```python
from build123d import *

# Parameters (mm, degrees)
BOSS_EXTRUDE1_DEPTH = 1.5
SKETCH2_W           = 28
SKETCH2_H           = 12.5
BOSS_EXTRUDE2_DEPTH = 8.5
SKETCH3_R           = 3
BOSS_EXTRUDE3_DEPTH = 4.5
SKETCH4_W           = 28
SKETCH4_H           = 12.5
BOSS_EXTRUDE4_DEPTH = 19.2
SKETCH5_W           = 3.625016777
SKETCH5_H           = 3.044537311
BOSS_EXTRUDE5_DEPTH = 12.5
BOSS_EXTRUDE7_DEPTH = 4


with BuildPart() as part:
    # Sketch1 → Boss-Extrude1 (new body)
    with BuildSketch(Plane(origin=(0, 0, 0), x_dir=(1, 0, 0), z_dir=(0, 1, 0))):
        with BuildLine():
            Line((20.25, -6.25), (-20.25, -6.25))
            Line((-20.25, -6.25), (-20.25, -1))
            Line((-20.25, -1), (-19.5, -1))
            ThreePointArc((-19.5, -1), (-15.234435563, 0), (-19.5, 1))
            Line((-19.5, 1), (-20.25, 1))
            Line((-20.25, 1), (-20.25, 6.25))
            Line((-20.25, 6.25), (20.25, 6.25))
            Line((20.25, 6.25), (20.25, 1))
            Line((20.25, 1), (19.5, 1))
            ThreePointArc((19.5, 1), (15.234435563, 0), (19.5, -1))
            Line((19.5, -1), (20.25, -1))
            Line((20.25, -1), (20.25, -6.25))
        make_face()
    extrude(amount=BOSS_EXTRUDE1_DEPTH)

    # Sketch2 → Boss-Extrude2 (add)
    with BuildSketch(Plane(origin=(0, 1.5, 0), x_dir=(1, 0, 0), z_dir=(0, 1, 0))):
        Rectangle(SKETCH2_W, SKETCH2_H)
    extrude(amount=BOSS_EXTRUDE2_DEPTH)

    # Sketch3 → Boss-Extrude3 (add)
    with BuildSketch(Plane(origin=(0, 10, 0), x_dir=(1, 0, 0), z_dir=(0, 1, 0))):
        with Locations((7, 0)):
            Circle(SKETCH3_R)
    extrude(amount=BOSS_EXTRUDE3_DEPTH)

    # Sketch4 → Boss-Extrude4 (add)
    with BuildSketch(Plane.XZ):
        Rectangle(SKETCH4_W, SKETCH4_H)
    extrude(amount=BOSS_EXTRUDE4_DEPTH)

    # Sketch5 → Boss-Extrude5 (add)
    with BuildSketch(Plane.XY.offset(6.25)):
        with Locations((15.812508389, -12.601527977)):
            Rectangle(SKETCH5_W, SKETCH5_H)
    extrude(amount=-BOSS_EXTRUDE5_DEPTH)

    # Sketch6 → Boss-Extrude7 (add)
    with BuildSketch(Plane(origin=(17.625016777, 0, 0), x_dir=(0, 0, -1), z_dir=(1, 0, 0))):
        with BuildLine():
            Line((-1.532511857, -12.7778257), (-1.512025454, -12.7778257))
            ThreePointArc((-1.512025454, -12.7778257), (0, -14.123796632), (1.512025454, -12.7778257))
            Line((1.512025454, -12.7778257), (1.532511857, -12.7778257))
            ThreePointArc((1.532511857, -12.7778257), (4.566805966, -12.601527977), (1.532511857, -12.425230254))
            Line((1.532511857, -12.425230254), (1.512025454, -12.425230254))
            ThreePointArc((1.512025454, -12.425230254), (0, -11.079259321), (-1.512025454, -12.425230254))
            Line((-1.512025454, -12.425230254), (-1.532511857, -12.425230254))
            ThreePointArc((-1.532511857, -12.425230254), (-4.566805966, -12.601527977), (-1.532511857, -12.7778257))
        make_face()
    extrude(amount=BOSS_EXTRUDE7_DEPTH)


solid = part.part
```
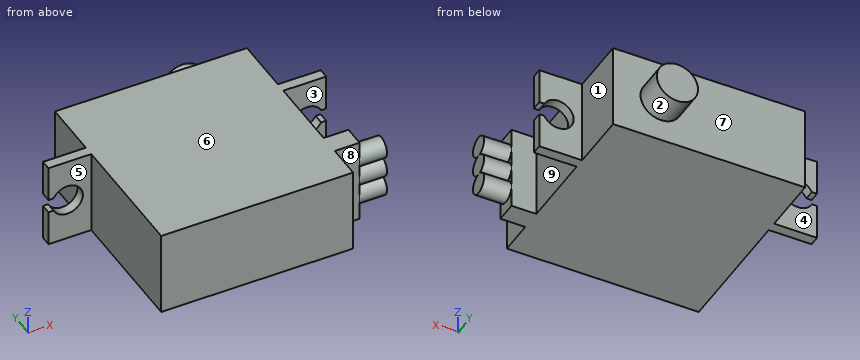
Part model, mm, in its own coordinate system. Face numbers are marked on the shaded views. A direction names the side the tool comes from. Coordinates: 2 decimals unless noted, no trailing zeros. Order: outer loops, then holes, each group sorted by start corner. A loop starts at its lowest first (then second) coordinate and runs counter-clockwise, first axis right, second up. Notation, with made-up numbers: (17.25, 23) -> (55.25, 23) arc R15 cw to (55.25, 42) -> close; hole circle Ø7 at (51.5, 89). An arc over 180 degrees is marked (long way). Put each result on its own line as item: value. Start each with the question number.
(1) Mould opens along Y. For the marked faces 6, 7, 8 and 9 say: pulls with the +Y half, pulls with the -Y half, needs draft (parallel to the pull), parting line crosses it, or undercut.
(2) Band-saw the part on A-A (x = -17.5). Give the cut face in (y, z), then the cut area to 3 significant figures.
(3) Band-saw the part on C-C (x = 17). Give the cut face in (y, z).
(4) Pin check, flat tips, straight feed: pin 1 Ø3 at (x, z) = (16, -3) entering from -Y; pin 2 Ø3 at (x, z) = (18.5, 0.5) entering from +Y; pin 3 Ø3 at (y, z) = (-2.5, -2.5) entering from +X. Stop position of each tip, or through.
(5) Probe line 1 along Y through (x, z) = (17, 5); line 2 along Y through (x, z) = (1, -4.5); line 3 along X through (y, z) = (8, -5). List the from-to ranges inside material, lowest first. Write a range as [from, to].
(6) Band-saw the part on B-B (x = 7). Give the cut face in (y, z), then the cut area to 3 significant figures.
(7) Which spindle directions (+Z, -Z, +X, -X, +Y, -Y) get a long thin tool onto all of the face, cutting with end or side? Do the marked faces 1, 2, 3, 4 and 5. Say none if no direction does.
(8) Band-saw the part on D-D (y = -8). Give the cut face in (x, z).
Determined:
1. face 6: needs draft
1. face 7: pulls with the +Y half
1. face 8: pulls with the -Y half
1. face 9: undercut
2. outline: (0, -6.25) -> (1.5, -6.25) -> (1.5, -2.25) -> (0, -2.25) -> close; (0, 2.25) -> (1.5, 2.25) -> (1.5, 6.25) -> (0, 6.25) -> close
2. area: 12.0 mm²
3. outline: (-14.12, -6.25) -> (-11.08, -6.25) -> (-11.08, 6.25) -> (-14.12, 6.25) -> close; (0, -6.25) -> (1.5, -6.25) -> (1.5, -2.2) -> (0, -2.2) -> close; (0, 2.2) -> (1.5, 2.2) -> (1.5, 6.25) -> (0, 6.25) -> close
4. pin 1: stops at y = -14.12
4. pin 2: stops at y = 1.5
4. pin 3: stops at x = 14
5. line 1: y = [-14.12, -11.08], [0, 1.5]
5. line 2: y = [-19.2, 10]
5. line 3: x = [-14, 14]
6. outline: (-19.2, -6.25) -> (10, -6.25) -> (10, -3) -> (14.5, -3) -> (14.5, 3) -> (10, 3) -> (10, 6.25) -> (-19.2, 6.25) -> close
6. area: 392 mm²
7. face 1: +Z, -Z, +X, +Y
7. face 2: +Y
7. face 3: +Z, -Z, +X
7. face 4: +Z, -Z, -X, +Y
7. face 5: +Z, -Z, -X, -Y
8. outline: (-14, -6.25) -> (14, -6.25) -> (14, 6.25) -> (-14, 6.25) -> close
